from build123d import *

# Parameters (mm, degrees)
F2_R     = 10
F3_DEPTH = 20.001
F4_R     = 21
F4_R_2   = 10
F5_DEPTH = 17


with BuildPart() as f1:
    # F0 (on Front) → F1 (revolve)
    with BuildSketch(Plane.XZ):
        with BuildLine():
            Line((0, 20), (0, 0))
            Line((0, 0), (50, 0))
            Line((50, 0), (50, 2))
            ThreePointArc((50, 2), (32.104477, 6.174129), (20, 20))
            Line((20, 20), (0, 20))
        make_face()
    revolve(axis=Axis((0, 0, 10), (0, 0, 1)))

    # F2 (on face) → F3 (cut, through all)
    with BuildSketch(Plane.XY.offset(20)):
        Circle(F2_R)
    extrude(amount=-F3_DEPTH, mode=Mode.SUBTRACT)

    # F4 (on face) → F5 (cut)
    with BuildSketch(Plane(origin=(0, 0, 0), x_dir=(1, 0, 0), z_dir=(0, 0, -1))):
        Circle(F4_R)
        Circle(F4_R_2, mode=Mode.SUBTRACT)
    extrude(amount=-F5_DEPTH, mode=Mode.SUBTRACT)


solid = f1.part
Here's how the part is built. I have some questions about the finished solid (model axes, mm). A direction names the side the tool comes from. Give positions to 0.01 mm unless a question says otherwise; leave off trailing zeros. Order: outer loops, then holes, each group sorted by start corner. A loop starts at its lowest first (then second) coordinate and runs counter-clockwise, first axis right, second up. Notation, with made-up numbers: (3, 29) -> (7, 29) arc R23 cw to (7, 55) -> close; hole circle Ø9 at (77, -38). An arc over 180 degrees is marked (long way). Use a Markdown table: item, result. Add a question column.
Item 1: If we mould it in two halves opening along X, with no side actions, what happens to faces 3 (the face through (-2.17, -9.76, 18.52)), 4 (the face through (-5, 9, 20)), 5 (the face through (47.69, 15.02, 1.01))? For each: pulls with the +X half, pulls with the -X half, needs draft (parallel to the pull), parting line crosses it, or undercut.
Item 2: I need wall thicknesses on line 1 (Y direction, x = -18, z = 14.5); line 2 (Y direction, x = -13.5, z = 10); line 3 (X direction, y = 0, z = 19). Which ranges of each line are inside material? Lowest first, please.
Item 3: Will these pins go through, and if not, where does the flat tip stop? pin 1 (25 mm diameter, centred on x = 0, y = 0, fed in from +Z); pin 2 (12 mm diameter, centred on y = 11, z = 5.5, fed in from -X); pin 3 (6 mm diameter, centred on y = 24.5, z = 4, fed in from -X); pin 4 (4 mm diameter, centred on x = -15.5, y = -7, fed in from -Z).
Item 4: For faces 1 (the face through (9, -5, 17)), 2 (the face through (1, -22, 0)), which set-ups out of +Z, -Z, +X, -X, +Y, -Y let a thin tool reach every point of the face, with its end or its side?
Item 5: Imagine slicing it at A-A on y = 0. Please give me the cut outline in (x, z), plus the area to 3 significant figures.
Item 6: Imagine slicing it at C-C on z = 8.25. Please give me the cut outline in (x, y), plus the area to 3 significant figures.
Data:
| question | item | result |
|---|---|---|
| 1 | face 3 | undercut |
| 1 | face 4 | needs draft |
| 1 | face 5 | parting line crosses it |
| 2 | line 1 | y = -14.48 to -10.82, 10.82 to 14.48 |
| 2 | line 2 | y = -23.42 to -16.09, 16.09 to 23.42 |
| 2 | line 3 | x = -20.45 to -10, 10 to 20.45 |
| 3 | pin 1 | stops at z = 20 |
| 3 | pin 2 | stops at x = -49.62 |
| 3 | pin 3 | stops at x = -44.77 |
| 3 | pin 4 | stops at z = 17 |
| 4 | face 1 | -Z |
| 4 | face 2 | -Z, +X, -X, +Y, -Y |
| 5 | outline | (-50, 0) -> (-21, 0) -> (-21, 17) -> (-10, 17) -> (-10, 20) -> (-20, 20) arc R30 cw to (-50, 2) -> close; (10, 17) -> (21, 17) -> (21, 0) -> (50, 0) -> (50, 2) arc R30 cw to (20, 20) -> (10, 20) -> close |
| 5 | area | 418 mm² |
| 6 | outline | circle Ø58.16 at (0, 0); hole circle Ø42 at (0, 0) |
| 6 | area | 1,270 mm² |
